from build123d import *

# Parameters (mm, degrees)
F0_R     = 2.75
F1_DEPTH = 2.45
F2_R     = 1.4
F3_DEPTH = 1.52
F4_R     = 0.915
F5_DEPTH = 1.52
F6_R     = 0.284492
F7_DEPTH = 0.92


with BuildPart() as f1:
    # F0 (on Right) → F1 (new body)
    with BuildSketch(Plane.YZ):
        Circle(F0_R)
    extrude(amount=F1_DEPTH)

    # F2 (on face) → F3 (join)
    with BuildSketch(Plane.YZ.offset(2.45)):
        Circle(F2_R)
    extrude(amount=F3_DEPTH)

    # F4 (on face) → F5 (join)
    with BuildSketch(Plane.YZ.offset(3.97)):
        Circle(F4_R)
    extrude(amount=F5_DEPTH)

    # F6 (on face) → F7 (join)
    with BuildSketch(Plane.YZ.offset(5.49)):
        Circle(F6_R)
    extrude(amount=F7_DEPTH)


solid = f1.part
Source: CAD feature listing. Evaluate the final solid. Frame: model axes, mm. A direction names the side the tool comes from. Give positions to 0.01 mm unless a question says otherwise; leave off trailing zeros. Order: outer loops, then holes, each group sorted by start corner. A loop starts at its lowest first (then second) coordinate and runs counter-clockwise, first axis right, second up. Notation, with made-up numbers: (30, -13) -> (65, -13) arc R21 ccw to (65, 1) -> close; hole circle Ø5 at (-27, -28). An arc over 180 degrees is marked (long way). Write item = value, one per line.
Q1. Cut plane C-C, the plane x = 1.5. Output: boundary loops of the cut face in (y, z).
Data:
outline = circle Ø5.5 at (0, 0)
Q2. Pin query (flat end, axial travel): pin 1 (1.5 mm diameter, centred on x = 1.5, z = 1, fed in from -Y); pin 2 (2 mm diameter, centred on x = 5, z = 1.5, fed in from -Y). Return the tip coordinate at first contact, or that it passes through.
Data:
pin_1 = -2.74
pin_2 = -0.77
Q3. Set-up query: faces 1 (the face through (5.49, 0.4, -0.2)), 2 (the face through (0, 0, 0)). Return all of +Z, -Z, +X, -X, +Y, -Y with unobstructed straight access to the full face (end or side cutting, diameter ignored); none if empty.
Data:
face_1 = +X
face_2 = +Z, -Z, -X, +Y, -Y
Q4. Material intervals for line 1 (X direction, y = -1.1, z = 0.45); line 2 (X direction, y = 1.8, z = 1.5); line 3 (Z direction, x = 2.25, y = -1.65), sorted ascending. Write a range as from..to.
Data:
line_1 = 0..3.97
line_2 = 0..2.45
line_3 = -2.2..2.2
Q5. Cut plane D-D, the plane y = -1.65. Output: boundary loops of the cut face in (x, z), and give its area (3 significant figures).
Data:
outline = (0, -2.2) -> (2.45, -2.2) -> (2.45, 2.2) -> (0, 2.2) -> close
area = 10.8 mm^2
